```python
from build123d import *

# Parameters (mm, degrees)
SKETCH_1_R      = 2.5
EXTRUDE_1_DEPTH = 200


with BuildPart() as part:
    # 草图1 → 凸台-拉伸1 (new body)
    with BuildSketch(Plane.XY):
        with BuildLine():
            Line((3.9, 0), (3.9, -2.010912703))
            ThreePointArc((3.9, -2.010912703), (4.052240935, -2.776279568), (4.485786438, -3.425126266))
            Line((4.485786438, -3.425126266), (6.560660172, -5.5))
            Line((6.560660172, -5.5), (7.9, -5.5))
            ThreePointArc((7.9, -5.5), (8.112132034, -5.412132034), (8.2, -5.2))
            Line((8.2, -5.2), (8.2, -3.4))
            ThreePointArc((8.2, -3.4), (8.287867966, -3.187867966), (8.5, -3.1))
            Line((8.5, -3.1), (9.2, -3.1))
            ThreePointArc((9.2, -3.1), (9.412132034, -3.187867966), (9.5, -3.4))
            Line((9.5, -3.4), (9.5, -3.6))
            Line((9.5, -3.6), (9.7, -3.6))
            ThreePointArc((9.7, -3.6), (9.912132034, -3.687867966), (10, -3.9))
            Line((10, -3.9), (10, -8.5))
            ThreePointArc((10, -8.5), (9.560660172, -9.560660172), (8.5, -10))
            Line((8.5, -10), (3.9, -10))
            ThreePointArc((3.9, -10), (3.687867966, -9.912132034), (3.6, -9.7))
            ThreePointArc((3.6, -9.7), (3.541421356, -9.558578644), (3.4, -9.5))
            ThreePointArc((3.4, -9.5), (3.187867966, -9.412132034), (3.1, -9.2))
            Line((3.1, -9.2), (3.1, -8.5))
            ThreePointArc((3.1, -8.5), (3.187867966, -8.287867966), (3.4, -8.2))
            Line((3.4, -8.2), (5.2, -8.2))
            ThreePointArc((5.2, -8.2), (5.412132034, -8.112132034), (5.5, -7.9))
            Line((5.5, -7.9), (5.5, -6.68492424))
            ThreePointArc((5.5, -6.68492424), (5.47716386, -6.570119211), (5.412132034, -6.472792206))
            Line((5.412132034, -6.472792206), (3.425126266, -4.485786438))
            ThreePointArc((3.425126266, -4.485786438), (2.776279568, -4.052240935), (2.010912703, -3.9))
            Line((2.010912703, -3.9), (0, -3.9))
            Line((0, -3.9), (-2.010912703, -3.9))
            ThreePointArc((-2.010912703, -3.9), (-2.776279568, -4.052240935), (-3.425126266, -4.485786438))
            Line((-3.425126266, -4.485786438), (-5.412132034, -6.472792206))
            ThreePointArc((-5.412132034, -6.472792206), (-5.47716386, -6.570119211), (-5.5, -6.68492424))
            Line((-5.5, -6.68492424), (-5.5, -7.9))
            ThreePointArc((-5.5, -7.9), (-5.412132034, -8.112132034), (-5.2, -8.2))
            Line((-5.2, -8.2), (-3.4, -8.2))
            ThreePointArc((-3.4, -8.2), (-3.187867966, -8.287867966), (-3.1, -8.5))
            Line((-3.1, -8.5), (-3.1, -9.2))
            ThreePointArc((-3.1, -9.2), (-3.187867966, -9.412132034), (-3.4, -9.5))
            ThreePointArc((-3.4, -9.5), (-3.541421356, -9.558578644), (-3.6, -9.7))
            ThreePointArc((-3.6, -9.7), (-3.687867966, -9.912132034), (-3.9, -10))
            Line((-3.9, -10), (-8.5, -10))
            ThreePointArc((-8.5, -10), (-9.560660172, -9.560660172), (-10, -8.5))
            Line((-10, -8.5), (-10, -3.9))
            ThreePointArc((-10, -3.9), (-9.912132034, -3.687867966), (-9.7, -3.6))
            Line((-9.7, -3.6), (-9.5, -3.6))
            Line((-9.5, -3.6), (-9.5, -3.4))
            ThreePointArc((-9.5, -3.4), (-9.412132034, -3.187867966), (-9.2, -3.1))
            Line((-9.2, -3.1), (-8.5, -3.1))
            ThreePointArc((-8.5, -3.1), (-8.287867965, -3.187867966), (-8.2, -3.4))
            Line((-8.2, -3.4), (-8.2, -5.2))
            ThreePointArc((-8.2, -5.2), (-8.112132034, -5.412132034), (-7.9, -5.5))
            Line((-7.9, -5.5), (-6.68492424, -5.5))
            ThreePointArc((-6.68492424, -5.5), (-6.570119211, -5.47716386), (-6.472792206, -5.412132034))
            Line((-6.472792206, -5.412132034), (-4.485786438, -3.425126266))
            ThreePointArc((-4.485786438, -3.425126266), (-4.052240935, -2.776279568), (-3.9, -2.010912703))
            Line((-3.9, -2.010912703), (-3.9, 0))
            Line((-3.9, 0), (-3.9, 2.010912703))
            ThreePointArc((-3.9, 2.010912703), (-4.052240935, 2.776279568), (-4.485786438, 3.425126266))
            Line((-4.485786438, 3.425126266), (-6.472792206, 5.412132034))
            ThreePointArc((-6.472792206, 5.412132034), (-6.570119211, 5.47716386), (-6.68492424, 5.5))
            Line((-6.68492424, 5.5), (-7.9, 5.5))
            ThreePointArc((-7.9, 5.5), (-8.112132034, 5.412132034), (-8.2, 5.2))
            Line((-8.2, 5.2), (-8.2, 3.4))
            ThreePointArc((-8.2, 3.4), (-8.287867965, 3.187867966), (-8.5, 3.1))
            Line((-8.5, 3.1), (-9.2, 3.1))
            ThreePointArc((-9.2, 3.1), (-9.412132034, 3.187867966), (-9.5, 3.4))
            Line((-9.5, 3.4), (-9.5, 3.6))
            Line((-9.5, 3.6), (-9.7, 3.6))
            ThreePointArc((-9.7, 3.6), (-9.912132034, 3.687867966), (-10, 3.9))
            Line((-10, 3.9), (-10, 8.5))
            ThreePointArc((-10, 8.5), (-9.560660172, 9.560660172), (-8.5, 10))
            Line((-8.5, 10), (-3.9, 10))
            ThreePointArc((-3.9, 10), (-3.687867966, 9.912132034), (-3.6, 9.7))
            Line((-3.6, 9.7), (-3.6, 9.5))
            Line((-3.6, 9.5), (-3.4, 9.5))
            ThreePointArc((-3.4, 9.5), (-3.187867966, 9.412132034), (-3.1, 9.2))
            Line((-3.1, 9.2), (-3.1, 8.5))
            ThreePointArc((-3.1, 8.5), (-3.187867966, 8.287867966), (-3.4, 8.2))
            Line((-3.4, 8.2), (-5.2, 8.2))
            ThreePointArc((-5.2, 8.2), (-5.412132034, 8.112132034), (-5.5, 7.9))
            Line((-5.5, 7.9), (-5.5, 6.68492424))
            ThreePointArc((-5.5, 6.68492424), (-5.47716386, 6.570119211), (-5.412132034, 6.472792206))
            Line((-5.412132034, 6.472792206), (-3.425126266, 4.485786438))
            ThreePointArc((-3.425126266, 4.485786438), (-2.776279568, 4.052240935), (-2.010912703, 3.9))
            Line((-2.010912703, 3.9), (0, 3.9))
            Line((0, 3.9), (2.010912703, 3.9))
            ThreePointArc((2.010912703, 3.9), (2.776279568, 4.052240935), (3.425126266, 4.485786438))
            Line((3.425126266, 4.485786438), (5.412132034, 6.472792206))
            ThreePointArc((5.412132034, 6.472792206), (5.47716386, 6.570119211), (5.5, 6.68492424))
            Line((5.5, 6.68492424), (5.5, 7.9))
            ThreePointArc((5.5, 7.9), (5.412132034, 8.112132034), (5.2, 8.2))
            Line((5.2, 8.2), (3.4, 8.2))
            ThreePointArc((3.4, 8.2), (3.187867966, 8.287867966), (3.1, 8.5))
            Line((3.1, 8.5), (3.1, 9.2))
            ThreePointArc((3.1, 9.2), (3.187867966, 9.412132034), (3.4, 9.5))
            Line((3.4, 9.5), (3.6, 9.5))
            Line((3.6, 9.5), (3.6, 9.7))
            ThreePointArc((3.6, 9.7), (3.687867966, 9.912132034), (3.9, 10))
            Line((3.9, 10), (8.5, 10))
            ThreePointArc((8.5, 10), (9.560660172, 9.560660172), (10, 8.5))
            Line((10, 8.5), (10, 3.9))
            ThreePointArc((10, 3.9), (9.912132034, 3.687867966), (9.7, 3.6))
            Line((9.7, 3.6), (9.5, 3.6))
            Line((9.5, 3.6), (9.5, 3.4))
            ThreePointArc((9.5, 3.4), (9.412132034, 3.187867966), (9.2, 3.1))
            Line((9.2, 3.1), (8.5, 3.1))
            ThreePointArc((8.5, 3.1), (8.287867966, 3.187867966), (8.2, 3.4))
            Line((8.2, 3.4), (8.2, 5.2))
            ThreePointArc((8.2, 5.2), (8.112132034, 5.412132034), (7.9, 5.5))
            Line((7.9, 5.5), (6.68492424, 5.5))
            ThreePointArc((6.68492424, 5.5), (6.570119211, 5.47716386), (6.472792206, 5.412132034))
            Line((6.472792206, 5.412132034), (4.485786438, 3.425126266))
            ThreePointArc((4.485786438, 3.425126266), (4.052240935, 2.776279568), (3.9, 2.010912703))
            Line((3.9, 2.010912703), (3.9, 0))
        make_face()
        Circle(SKETCH_1_R, mode=Mode.SUBTRACT)
    extrude(amount=EXTRUDE_1_DEPTH)


solid = part.part
```
Geometry check sheet. Reference: the model listing, model coordinates, mm. A direction names the side the tool comes from. Round coordinates to 2 decimals unless told otherwise and drop trailing zeros. Order: outer loops, then holes, each group sorted by start corner. A loop starts at its lowest first (then second) coordinate and runs counter-clockwise, first axis right, second up. Notation, with made-up numbers: (-18.75, 14) - (28.25, 14) arc R28 ccw to (28.25, 38) - close; hole circle Ø2 at (69, 42). An arc over 180 degrees is marked (long way). Use a Markdown table: item, result. Add a question column.
1) Set-up check for faces 4 (the flat face through (0, -3.9, 99)), 5 (the flat face through (-3.9, 0, 99)), 6 (the flat face through (3.9, 0, 99)): record each of +Z, -Z, +X, -X, +Y, -Y from which the full face is reachable in a straight line by a thin tool's end or side.
2) Section check A-A (x = 0). Record the cut outline in (y, z).
3) Thickness scan on line 1 along Y through (x, z) = (0, 138); line 2 along X through (y, z) = (-8.5, 12); line 3 along X through (y, z) = (8, 48). Record the ranges inside material, lowest first.
4) Mould release check, pull along X, two halves, no side actions. Record for faces 1 (the flat face through (0, 3.9, 99)), 2 (the flat face through (-10, 6, 99)), 3 (the flat face through (-6, -10, 99)): released by +X, released by -X, zero draft, split by the parting line, or undercut.
5) Gauge pin test, flat ends, axial feed: P1, Ø5, axis at x = -4.5, y = -1, coming from the +Z side; P2, Ø1.5, axis at y = 1.5, z = 115, coming from the +X side; P3, Ø0.8, axis at x = 9, z = 53.5, coming from the +Y side; P4, Ø2, axis at x = -0.5, y = -7.5, coming from the +Z side. Record the tip position at first contact, or that the pin passes through.
Established:
| question | item | result |
|---|---|---|
| 1 | face 4 | +Z, -Z, -Y |
| 1 | face 5 | +Z, -Z, -X |
| 1 | face 6 | +Z, -Z, +X |
| 2 | outline | (-3.9, 0) - (-2.5, 0) - (-2.5, 200) - (-3.9, 200) - close; (2.5, 0) - (3.9, 0) - (3.9, 200) - (2.5, 200) - close |
| 3 | line 1 | -3.9 to -2.5, 2.5 to 3.9 |
| 3 | line 2 | -10 to -3.1, 3.1 to 10 |
| 3 | line 3 | -10 to -5.48, 5.48 to 10 |
| 4 | face 1 | undercut |
| 4 | face 2 | released by -X |
| 4 | face 3 | zero draft |
| 5 | P1 | z = 200 |
| 5 | P2 | x = 3.91 |
| 5 | P3 | y = 10 |
| 5 | P4 | through |
